Geometry: final body of the model. Coordinates: model frame, mm. Coordinates: 2 decimals unless noted, no trailing zeros. Loops run counter-clockwise (first coordinate to the right, second up) from the corner with the lowest first, then second, coordinate; pieces in that order, holes last. Notation, with made-up numbers: (37.25, -39.75) - (79.25, -39.75) arc R10 cw to (79.25, -31.75) - close; hole circle Ø6 at (-27.5, 49). An arc over 180 degrees is marked (long way). Put each result on its own line as item: value. Start each with the question number.
1) Material intervals for line 1 along Y through (x, z) = (307, 1.35); line 2 along X through (y, z) = (5.75, 0.65); line 3 along Y through (x, z) = (339.5, 1.8), sorted ascending. Write a range as from..to.
2) Section A-A on z = 2.35. Count the separate pieces of the cut face and the enclosed holes in it, and give its area (3 significant figures).
3) Section B-B on x = 347. Output: boundary loops of the cut face in (y, z), and give its area (3 significant figures).
4) Contact query for a flat-ended pin moving along its axis: pin 1 Ø1.5 at (x, z) = (186, 1.5) entering from +Y. Output: stop coordinate, or through.
Autodesk Inventor part; units mm, degrees
ref_plane "YZ Plane" through (0, 0, 0) normal (1, 0, 0) x (0, 1, 0)
ref_plane "XZ Plane" through (0, 0, 0) normal (0, 1, 0) x (-1, 0, 0)
ref_plane "XY Plane" through (0, 0, 0) normal (0, 0, 1) x (1, 0, 0)
sketch "Szkic1" plane through (0, 0, 0) normal (0, 0, 1) x (1, 0, 0)
  line L0 (444.7232, 18.712) -> (444.7232, -11.288)
  line L1 (444.7232, -11.288) -> (-15.2768, -11.288)
  line L2 (-15.2768, -11.288) -> (-15.2768, 18.712)
  line L3 (-15.2768, 18.712) -> (36.1232, 18.712)
  line L4 (36.1232, 18.712) -> (36.1232, 17.712)
  line L5 (36.1232, 17.712) -> (393.3232, 17.712)
  line L6 (393.3232, 17.712) -> (393.3232, 18.712)
  line L7 (393.3232, 18.712) -> (444.7232, 18.712)
  point P0 (0, 0)
  dimension "d0" = 460
  dimension "d1" = 30
  dimension "d2" = 1
  dimension "d3" = 51.4
  dimension "d4" = 51.4
extrude "Wyciągnięcie proste1" add sketch "Szkic1" along normal blind 3
chamfer "Faza1" distance 10 distance2 1 1 edges at (36.1232, 17.712, 1.5) measured on face at (274.2565, 17.712, 1)
chamfer "Faza2" distance 10 distance2 1 1 edges at (393.3232, 17.712, 1.5) measured on face at (277.5897, 17.712, 1)
fillet "Zaokrąglenie1" radius 5 2 edges at (444.7232, 18.712, 1.5) (-15.2768, 18.712, 1.5)
chamfer "Faza3" distance 40 distance2 15 1 edges at (444.7232, -11.288, 1.5) measured on face at (138.0565, -11.288, 1)
chamfer "Faza4" distance 40 distance2 15 1 edges at (-15.2768, -11.288, 1.5) measured on face at (124.7232, -11.288, 2)
sketch "Szkic2" plane through (0, 0, 3) normal (0, 0, 1) x (1, 0, 0)
  line L0 (383.3232, 17.712) -> (46.1232, 17.712)
  line L1 (-15.2768, 13.712) -> (-15.2768, 3.712)
  line L2 (444.7232, 3.712) -> (444.7232, 13.712)
  line L3 (36.1232, 18.712) -> (-10.2768, 18.712)
  line L4 (439.7232, 18.712) -> (393.3232, 18.712)
  point P0 (0, 0)
  point P1 (34.7232, 4.712)
  point P2 (394.7232, 4.712)
  point P3 (109.7232, 4.712)
  point P4 (319.7232, 4.712)
  dimension "d34" = 50
  dimension "d35" = 75
  dimension "d36" = 75
  dimension "d37" = 50
  dimension "d39" = 14
  dimension "d40" = 14
  dimension "d41" = 14
  dimension "d42" = 14
fillet "Zaokrąglenie2" radius 3 4 edges at (444.7232, 3.712, 1.5) (404.7232, -11.288, 1.5) (24.7232, -11.288, 1.5) (-15.2768, 3.712, 1.5)
hole "Otwór1" at (34.7232, 4.712, 3) at (394.7232, 4.712, 3) at (109.7232, 4.712, 3) at (319.7232, 4.712, 3) direction (0, 0, -1) diameter 3 end through all
sketch "Szkic4" plane through (0, 0, 0) normal (0, 0, -1) x (-1, 0, 0)
  circle A0 centre (-109.7232, 4.712) radius 1.5
  circle A1 centre (-34.7232, 4.712) radius 1.5
  circle A2 centre (-394.7232, 4.712) radius 1.5
  circle A3 centre (-319.7232, 4.712) radius 1.5
  arc A4 (13.3302, 2.9821) -> (15.2768, 5.791) centre (12.2768, 5.791) ccw
  line L0 (15.2768, 13.712) -> (15.2768, 5.791)
  arc A5 (15.2768, 13.712) -> (10.2768, 18.712) centre (10.2768, 13.712) ccw
  line L1 (-36.1232, 18.712) -> (10.2768, 18.712)
  line L2 (-46.1232, 17.712) -> (-36.1232, 18.712)
  line L3 (-383.3232, 17.712) -> (-46.1232, 17.712)
  line L4 (-393.3232, 18.712) -> (-383.3232, 17.712)
  line L5 (-439.7232, 18.712) -> (-393.3232, 18.712)
  arc A6 (-439.7232, 18.712) -> (-444.7232, 13.712) centre (-439.7232, 13.712) ccw
  line L6 (-444.7232, 5.791) -> (-444.7232, 13.712)
  arc A7 (-444.7232, 5.791) -> (-442.7766, 2.9821) centre (-441.7232, 5.791) ccw
  line L7 (-405.2326, -11.0969) -> (-442.7766, 2.9821)
  arc A8 (-405.2326, -11.0969) -> (-404.1792, -11.288) centre (-404.1792, -8.288) ccw
  line L8 (-25.2672, -11.288) -> (-404.1792, -11.288)
  arc A9 (-25.2672, -11.288) -> (-24.2138, -11.0969) centre (-25.2672, -8.288) ccw
  line L9 (13.3302, 2.9821) -> (-24.2138, -11.0969)
  line L10 (-292.2232, 13.612) -> (-12.8371, 13.612) construction
  line L11 (-12.8371, 13.612) -> (-12.8371, -7.1032) construction
  line L12 (-12.8371, -7.1032) -> (-292.2232, -7.1032) construction
  line L13 (-292.2232, -7.1032) -> (-292.2232, 13.612) construction
  point P0 (0, 0)
  dimension "d43" = 4.1
  dimension "d44" = 152.5
extrude "Wyciągnięcie proste3" [suppressed]
sketch "Szkic5" plane through (0, 0, 0) normal (0, 0, -1) x (-1, 0, 0)
  arc A0 (13.3302, 2.9821) -> (15.2768, 5.791) centre (12.2768, 5.791) ccw
  line L0 (15.2768, 13.712) -> (15.2768, 5.791)
  arc A1 (15.2768, 13.712) -> (10.2768, 18.712) centre (10.2768, 13.712) ccw
  line L1 (-36.1232, 18.712) -> (10.2768, 18.712)
  line L2 (-46.1232, 17.712) -> (-36.1232, 18.712)
  line L3 (-383.3232, 17.712) -> (-46.1232, 17.712)
  line L4 (-393.3232, 18.712) -> (-383.3232, 17.712)
  line L5 (-439.7232, 18.712) -> (-393.3232, 18.712)
  arc A2 (-439.7232, 18.712) -> (-444.7232, 13.712) centre (-439.7232, 13.712) ccw
  line L6 (-444.7232, 5.791) -> (-444.7232, 13.712)
  arc A3 (-444.7232, 5.791) -> (-442.7766, 2.9821) centre (-441.7232, 5.791) ccw
  line L7 (-405.2326, -11.0969) -> (-442.7766, 2.9821)
  arc A4 (-405.2326, -11.0969) -> (-404.1792, -11.288) centre (-404.1792, -8.288) ccw
  line L8 (-25.2672, -11.288) -> (-404.1792, -11.288)
  arc A5 (-25.2672, -11.288) -> (-24.2138, -11.0969) centre (-25.2672, -8.288) ccw
  line L9 (13.3302, 2.9821) -> (-24.2138, -11.0969)
  circle A6 centre (-319.7232, 4.712) radius 1.5
  circle A7 centre (-394.7232, 4.712) radius 1.5
  circle A8 centre (-34.7232, 4.712) radius 1.5
  circle A9 centre (-109.7232, 4.712) radius 1.5
  line L10 (-436.9348, 14.712) -> (34.576, 14.712)
  line L11 (-429.8152, 7.212) -> (-144.7013, 7.212)
  line L12 (-310.7232, 7.212) -> (-305.7232, 7.212)
  line L13 (-305.7232, 7.212) -> (-305.7232, -7.788)
  line L14 (-305.7232, -7.788) -> (-310.7232, -7.788)
  line L15 (-310.7232, -7.788) -> (-310.7232, 7.212)
  line L16 (-428.7978, 2.212) -> (-310.7232, 2.212)
  line L17 (-305.7232, 2.212) -> (-143.684, 2.212)
  line L18 (-434.2328, -5.288) -> (-310.7232, -5.288)
  line L19 (-305.7232, -5.288) -> (47.3582, -5.288)
  point P0 (0, 0)
  dimension "d47" = 3
  dimension "d49" = 2.5
  dimension "d51" = 5
  dimension "d52" = 15
  dimension "d54" = 9
extrude "Wyciągnięcie proste4" cut sketch "Szkic5" against normal through all contours L13 L14 L15 L11
fillet "Zaokrąglenie3" radius 1 4 edges at (305.7232, -7.788, 1.5) (310.7232, -7.788, 1.5) (310.7232, 7.212, 1.5) (305.7232, 7.212, 1.5)
equation "\"d4\" = d3"
properties part number "LC_PLEXI_3mm_Heatbed_Platform_Logo_Plate_Diffuser"
Answer block:
1. line 1: y = -11.29..-7.79, 7.21..17.71
1. line 2: x = -15.28..33.64, 35.81..108.64, 110.81..305.72, 310.72..318.64, 320.81..393.64, 395.81..444.72
1. line 3: y = -11.29..17.71
2. separate pieces: 1
2. enclosed holes: 5
2. area: 12,700 mm²
3. outline: (-11.29, 0) - (17.71, 0) - (17.71, 3) - (-11.29, 3) - close
3. area: 87.0 mm²
4. pin 1: stops at y = 17.71
